from build123d import *

# Parameters (mm, degrees)
BOSS_EXTRUDE1_DEPTH = 198
SHELL1_T            = -7
BOSS_EXTRUDE2_DEPTH = 191
SKETCH3_W           = 95.245639834
SKETCH3_H           = 3
BOSS_EXTRUDE3_DEPTH = 191
SKETCH4_R           = 1.585
CUT_EXTRUDE1_DEPTH  = 5
BOSS_EXTRUDE4_DEPTH = 25


with BuildPart() as part:
    # Sketch1 → Boss-Extrude1 (new body)
    with BuildSketch(Plane(origin=(0, 0, 0), x_dir=(0, 0, -1), z_dir=(1, 0, 0))):
        Polygon((22.10846405, 0), (32.441807929, 17.899216821), (45.200737204, 39.99998538), (121.214199537, 39.99998538), (121.18, 0), align=None)
    extrude(amount=BOSS_EXTRUDE1_DEPTH)

    # Shell1
    shell1_openings = [part.faces().sort_by_distance(p)[0] for p in [
        (99, 0, -71.644232025),
    ]]
    offset(amount=SHELL1_T, openings=shell1_openings, kind=Kind.INTERSECTION)

    # Sketch2 → Boss-Extrude2 (add)
    with BuildSketch(Plane.ZY):
        Polygon((-30.191216521, 0), (-32.974854852, 0), (-52.025978727, 32.99998538), (-49.242340395, 32.99998538), align=None)
    extrude(amount=-BOSS_EXTRUDE2_DEPTH)

    # Sketch3 → Boss-Extrude3 (add)
    with BuildSketch(Plane.ZY):
        with Locations((-73.557180083, 1.5)):
            Rectangle(SKETCH3_W, SKETCH3_H)
    extrude(amount=-BOSS_EXTRUDE3_DEPTH)

    # Sketch4 → Cut-Extrude1 (cut)
    with BuildSketch(Plane(origin=(0, 3, 0), x_dir=(1, 0, 0), z_dir=(0, 1, 0))):
        with Locations(Location((11, 109.182562408, 0), (0, 0, 270))):
            Circle(SKETCH4_R)
        with Locations(Location((11, 39.706775972, 0), (0, 0, 270))):
            Circle(SKETCH4_R)
    cut_extrude1 = extrude(amount=-CUT_EXTRUDE1_DEPTH, mode=Mode.SUBTRACT)

    # Mirror1: Cut-Extrude1 across plane
    add(cut_extrude1.mirror(Plane(origin=(99, 0, 0), x_dir=(0, 0, 1), z_dir=(1, 0, 0))), mode=Mode.SUBTRACT)

    # Sketch5 → Boss-Extrude4 (add)
    with BuildSketch(Plane(origin=(0, 3, 0), x_dir=(1, 0, 0), z_dir=(0, 1, 0))):
        Polygon((187.246573538, 56.499587918), (77.246576653, 56.473406784), (77.260934082, 91.473403839), (187.260930967, 91.499584973), align=None)
    extrude(amount=BOSS_EXTRUDE4_DEPTH)


solid = part.part
The model under review builds one solid part; all positions refer to its coordinate system, in mm. A direction names the side the tool comes from. Give positions to 0.01 mm unless a question says otherwise; leave off trailing zeros. Order: outer loops, then holes, each group sorted by start corner. A loop starts at its lowest first (then second) coordinate and runs counter-clockwise, first axis right, second up. Notation, with made-up numbers: M 52,26 L 70,26 A36 ccw 70,61 Z; hole C -26.5,59 d2. An arc over 180 degrees is marked long. Answer in a Markdown table with one row per item. Add a question column.
1. For pin 1 Ø15 at (y, z) = (12.5, -67.5) entering from -X; pin 2 Ø12 at (x, y) = (151.5, 9.5) entering from -Z; pin 3 Ø3 at (x, z) = (187, -109.18) entering from -Y; pin 4 Ø3.5 at (x, z) = (187, -39.71) entering from +Y, all flat-tipped, find the tip position at first contact; note any pin that passes through.
2. Machinability: for faces 4 (the flat face through (77, 3, -93)), 5 (the flat face through (98, 40, -83)), which of the approach directions +Z, -Z, +X, -X, +Y, -Y give a long, thin tool a straight path to every point of the face, cutting with its end or side? Answer none if there is none.
3. Mouldability with a two-part tool opening along X and no side actions: class faces 1 (the flat face through (198, 20, -72)), 2 (the flat face through (0, 20, -82)), 3 (the flat face through (191, 18, -75)) as released by +X, released by -X, zero draft, split by the parting line, or undercut.
4. To check wall thickness, follow line 1 along X through (y, z) = (20, -57); line 2 along X through (y, z) = (21.5, -88); line 3 along X through (y, z) = (6, -39.5). State the ranges of each line that lie inside material, in increasing order.
5. Add section B-B on z = -97. State the section outline as (x, y) points, plus the area to 3 significant figures.
6. Add section A-A on x = 50. State the section outline as (y, z) points.
7. Add section D-D on x = 181.5. State the section outline as (y, z) points.
8. Add section C-C on y = 10. State the section outline as (x, z) points.
The answers:
| question | item | result |
|---|---|---|
| 1 | pin 1 | x = 0 |
| 1 | pin 2 | z = -121.19 |
| 1 | pin 3 | y = 33 |
| 1 | pin 4 | y = 33.52 |
| 2 | face 4 | none |
| 2 | face 5 | +Z, -Z, +X, -X, +Y |
| 3 | face 1 | released by +X |
| 3 | face 2 | released by -X |
| 3 | face 3 | undercut |
| 4 | line 1 | 0 to 7, 77.25 to 187.25, 191 to 198 |
| 4 | line 2 | 0 to 7, 77.26 to 187.26, 191 to 198 |
| 4 | line 3 | 0 to 7, 191 to 198 |
| 5 | outline | M 0,0 L 198,0 L 198,40 L 0,40 Z; hole M 7,3 L 191,3 L 191,33 L 7,33 Z |
| 5 | area | 2,400 mm2 |
| 6 | outline | M 0,-121.18 L 40,-121.21 L 40,-45.2 L 0,-22.11 Z; hole M 3,-114.18 L 33,-114.21 L 33,-52.03 L 3,-34.71 Z |
| 7 | outline | M 0,-121.18 L 40,-121.21 L 40,-45.2 L 0,-22.11 Z; hole M 3,-114.18 L 33,-114.21 L 33,-52.03 L 3,-34.71 L 3,-56.5 L 28,-56.5 L 28,-91.5 L 3,-91.5 Z |
| 8 | outline | M 0,-121.19 L 198,-121.19 L 198,-27.88 L 0,-27.88 Z; M 77.25,-56.47 L 77.26,-91.47 L 187.26,-91.5 L 187.25,-56.5 Z; hole M 7,-114.19 L 191,-114.19 L 191,-38.75 L 7,-38.75 Z |
